from build123d import *

# Parameters (mm, degrees)
F0_W     = 28.5
F0_H     = 21.5
F1_DEPTH = 1.2
F2_W     = 28.5
F2_H     = 21.5
F3_DEPTH = 6
F5_DEPTH = 2
F6_W     = 22
F6_H     = 6
F7_DEPTH = 3.25
F8_R     = 1.6
F9_DEPTH = 2


with BuildPart() as f1:
    # F0 (on Top) → F1 (new body)
    with BuildSketch(Plane.XY):
        with BuildLine():
            ThreePointArc((18.95, 11.7), (17.192641, 15.942641), (12.95, 17.7))
            Line((12.95, 17.7), (-12.95, 17.7))
            ThreePointArc((-12.95, 17.7), (-17.192641, 15.942641), (-18.95, 11.7))
            Line((-18.95, 11.7), (-18.95, -11.7))
            ThreePointArc((-18.95, -11.7), (-17.192641, -15.942641), (-12.95, -17.7))
            Line((-12.95, -17.7), (12.95, -17.7))
            ThreePointArc((12.95, -17.7), (17.192641, -15.942641), (18.95, -11.7))
            Line((18.95, -11.7), (18.95, 11.7))
        make_face()
        Rectangle(F0_W, F0_H, mode=Mode.SUBTRACT)
    extrude(amount=F1_DEPTH)

    # F2 (on face) → F3 (join)
    with BuildSketch(Plane.XY.offset(1.2)):
        with BuildLine():
            ThreePointArc((17.5, 11), (16.035534, 14.535534), (12.5, 16))
            Line((12.5, 16), (-12.5, 16))
            ThreePointArc((-12.5, 16), (-16.035534, 14.535534), (-17.5, 11))
            Line((-17.5, 11), (-17.5, -11))
            ThreePointArc((-17.5, -11), (-16.035534, -14.535534), (-12.5, -16))
            Line((-12.5, -16), (12.5, -16))
            ThreePointArc((12.5, -16), (16.035534, -14.535534), (17.5, -11))
            Line((17.5, -11), (17.5, 11))
        make_face()
        Rectangle(F2_W, F2_H, mode=Mode.SUBTRACT)
    extrude(amount=F3_DEPTH)

    # F4 (on face) → F5 (join)
    with BuildSketch(Plane.XY.offset(7.2)):
        with BuildLine():
            ThreePointArc((17.5, 11), (16.035534, 14.535534), (12.5, 16))
            Line((12.5, 16), (-12.5, 16))
            ThreePointArc((-12.5, 16), (-16.035534, 14.535534), (-17.5, 11))
            Line((-17.5, 11), (-17.5, -11))
            ThreePointArc((-17.5, -11), (-16.035534, -14.535534), (-12.5, -16))
            Line((-12.5, -16), (12.5, -16))
            ThreePointArc((12.5, -16), (16.035534, -14.535534), (17.5, -11))
            Line((17.5, -11), (17.5, 11))
        make_face()
    extrude(amount=F5_DEPTH)

    # F6 (on face) → F7 (cut, through all)
    with BuildSketch(Plane(origin=(-17.5, 0, 0), x_dir=(0, -1, 0), z_dir=(-1, 0, 0))):
        with Locations((0, 4.2)):
            Rectangle(F6_W, F6_H)
    extrude(amount=-F7_DEPTH, mode=Mode.SUBTRACT)

    # F8 (on face) → F9 (cut, through all)
    with BuildSketch(Plane.XY.offset(9.2)):
        with Locations((10, 6)):
            Circle(F8_R)
        with Locations((10, -6)):
            Circle(F8_R)
    extrude(amount=-F9_DEPTH, mode=Mode.SUBTRACT)


solid = f1.part
Here's how the part is built. I have some questions about the finished solid (model axes, mm). A direction names the side the tool comes from. Round coordinates to 2 decimals unless told otherwise and drop trailing zeros. Loops run counter-clockwise (first coordinate to the right, second up) from the corner with the lowest first, then second, coordinate; pieces in that order, holes last. Notation, with made-up numbers: (-18.5, 44.5) - (-12.5, 44.5) arc R13 cw to (-12.5, 69.5) - close; hole circle Ø11 at (-29.5, 83). An arc over 180 degrees is marked (long way). One line per question, with ' | ' between items. Start each with the question number.
Q1. Will these pins go through, and if not, where does the flat tip stop? pin 1 (1.5 mm diameter, centred on x = -0.5, z = 2, fed in from -Y); pin 2 (6 mm diameter, centred on x = 8, y = -4.5, fed in from -Z); pin 3 (1 mm diameter, centred on x = -3.5, z = 7.5, fed in from +Y); pin 4 (3 mm diameter, centred on x = 10, y = -6, fed in from -Z).
Q2. Please list where these lines run through material, in increasing order: line 1 (Y direction, x = 10, z = 7.7); line 2 (Y direction, x = 2.5, z = 3.5); line 3 (Z direction, x = -10.5, y = 5.5). Write a range as [from, to].
Q3. I want a section at A-A (y = 2). Write out the boundary of the cut face in (x, z).
Q4. I want a section at B-B (x = 10). Write out the boundary of the cut face in (y, z), then the cut area to 3 significant figures.
Q5. We'd pull the mould along X, two halves only. Please class faces 6 (the cylindrical face through (8.4, -5.93, 8.21)), 7 (the cylindrical face through (17.146, -15.989, 0.592)), 8 (the flat face through (-17.5, 0, 8)): +X half, -X half, draft (parallel to the pull), parting line (faces both ways), or undercut.
Q6. For faces 1 (the flat face through (0, -16, 5)), 2 (the flat face through (0, 16, 5)), 3 (the flat face through (14.25, 0, 4)), 4 (the cylindrical face through (-16.07, -14.5, 5.14)), 5 (the flat face through (17.5, 0, 5)), which set-ups out of +Z, -Z, +X, -X, +Y, -Y let a thin tool reach every point of the face, with its end or its side?
Q7. I want a section at D-D (z = 8.5). Write out the boundary of the cut face in (x, y), then the cut area to 3 significant figures.
Q8. I want a section at C-C (y = 6). Write out the boundary of the cut face in (x, z).
Response values:
1) pin 1: stops at y = -16 | pin 2: stops at z = 7.2 | pin 3: stops at y = 16 | pin 4: passes through
2) line 1: y = [-16, -7.6], [-4.4, 4.4], [7.6, 16] | line 2: y = [-16, -10.75], [10.75, 16] | line 3: z = [7.2, 9.2]
3) outline: (-18.95, 0) - (-14.25, 0) - (-14.25, 1.2) - (-18.95, 1.2) - close; (-17.5, 7.2) - (14.25, 7.2) - (14.25, 0) - (18.95, 0) - (18.95, 1.2) - (17.5, 1.2) - (17.5, 9.2) - (-17.5, 9.2) - close
4) outline: (-17.7, 0) - (-10.75, 0) - (-10.75, 7.2) - (-7.6, 7.2) - (-7.6, 9.2) - (-16, 9.2) - (-16, 1.2) - (-17.7, 1.2) - close; (-4.4, 7.2) - (4.4, 7.2) - (4.4, 9.2) - (-4.4, 9.2) - close; (7.6, 7.2) - (10.75, 7.2) - (10.75, 0) - (17.7, 0) - (17.7, 1.2) - (16, 1.2) - (16, 9.2) - (7.6, 9.2) - close | area: 131 mm²
5) face 6: undercut | face 7: +X half | face 8: -X half
6) face 1: +Z, +X, -X, -Y | face 2: +Z, +X, -X, +Y | face 3: -Z | face 4: +Z, -X, -Y | face 5: +Z, +X, +Y, -Y
7) outline: (-17.5, -11) arc R5 ccw to (-12.5, -16) - (12.5, -16) arc R5 ccw to (17.5, -11) - (17.5, 11) arc R5 ccw to (12.5, 16) - (-12.5, 16) arc R5 ccw to (-17.5, 11) - close; hole circle Ø3.2 at (10, -6); hole circle Ø3.2 at (10, 6) | area: 1,080 mm²
8) outline: (-18.95, 0) - (-14.25, 0) - (-14.25, 1.2) - (-18.95, 1.2) - close; (-17.5, 7.2) - (8.4, 7.2) - (8.4, 9.2) - (-17.5, 9.2) - close; (11.6, 7.2) - (14.25, 7.2) - (14.25, 0) - (18.95, 0) - (18.95, 1.2) - (17.5, 1.2) - (17.5, 9.2) - (11.6, 9.2) - close
